Can you work these out from the model? Positions are in its coordinate system, mm. A direction names the side the tool comes from. Round coordinates to 2 decimals unless told otherwise and drop trailing zeros. Write each loop counter-clockwise with the first axis right and the second up, starting at its lowest first coordinate (ties: lowest second). Pieces come first, ordered by that corner, then holes. Notation, with made-up numbers: M -30.5,29 L -0.5,29 A26 ccw -0.5,57 Z; hole C 40,41.25 d9. An arc over 180 degrees is marked long. Answer as a JSON object with one key per item and string values. Group by question number.
1) Suppose I cut it at C-C, the plane y = 19. Write out the boundary of the cut face in (x, z).
2) Suppose I cut it at D-D, the plane x = 206. Write out the boundary of the cut face in (y, z).
3) I'm going to push flat-ended pins straight in: pin 1 Ø6 at (y, z) = (6, -75) entering from -X; pin 2 Ø8 at (x, y) = (156, 4) entering from +Z. Where does each tip first touch, or does it pass through?
4) Please list where these lines run through material, in increasing order: L1, parallel to X at y = 7.75, z = -46; L2, parallel to Z at x = 6.5, y = 6; L3, parallel to Y at x = 6, z = -75. Write a range as [from, to].
5) On a 3-axis mill with a long thin cutter (end or side, diameter ignored), from which of +Z, -Z, +X, -X, +Y, -Y can I reach the whole of each face in a straight line? I mean faces 1 (the flat face through (109, 11, -141)), 2 (the flat face through (109, 26, -121.5)), 3 (the flat face through (109, 28.67, -123)). Say none if no direction works.
6) Suppose I cut it at A-A, the plane x = 70. Write out the boundary of the cut face in (y, z).
7) Suppose I cut it at B-B, the plane z = -100. Write out the boundary of the cut face in (x, y), and give its area (3 significant figures).
8) If we mould it in two halves opening along Z, with no side actions, what happens to faces 4 (the flat face through (109, 12, -150)), 5 (the flat face through (0, 12, -72)), 6 (the flat face through (109, 23, 0)), 7 (the flat face through (193.5, 26, -70))? For each: +Z half, -Z half, draft (parallel to the pull), parting line (faces both ways), or undercut.
from build123d import *

# Parameters (mm, degrees)
BOSS_EXTRUDE1_DEPTH                               = 22.59
SKETCH2_W                                         = 220
SKETCH2_H                                         = 150
SKETCH2_W_2                                       = 167
SKETCH2_H_2                                       = 102
BOSS_EXTRUDE2_DEPTH                               = 6.08
CSK_FOR_6_FLAT_HEAD_SOCKET_CAP_SCREW2_D           = 3.7973
CSK_FOR_6_FLAT_HEAD_SOCKET_CAP_SCREW2_DEPTH       = 9
CSK_FOR_6_FLAT_HEAD_SOCKET_CAP_SCREW2_CSINK_D     = 7.7978
CSK_FOR_6_FLAT_HEAD_SOCKET_CAP_SCREW2_CSINK_ANGLE = 82
CSK_FOR_6_FLAT_HEAD_SOCKET_CAP_SCREW3_D           = 3.7973
CSK_FOR_6_FLAT_HEAD_SOCKET_CAP_SCREW3_CSINK_D     = 7.7978
CSK_FOR_6_FLAT_HEAD_SOCKET_CAP_SCREW3_CSINK_ANGLE = 82
CSK_FOR_6_FLAT_HEAD_SOCKET_CAP_SCREW4_D           = 3.7973
CSK_FOR_6_FLAT_HEAD_SOCKET_CAP_SCREW4_CSINK_D     = 7.7978
CSK_FOR_6_FLAT_HEAD_SOCKET_CAP_SCREW4_CSINK_ANGLE = 82
FILLET1_R                                         = 4


with BuildPart() as part:
    # Sketch1 → Boss-Extrude1 (new body)
    with BuildSketch(Plane(origin=(0, 0, 0), x_dir=(1, 0, 0), z_dir=(0, 1, 0))):
        Polygon((211, 0), (220, 0), (220, 150), (0, 150), (0, 0), (9, 0), (9, 141), (211, 141), align=None)
    extrude(amount=BOSS_EXTRUDE1_DEPTH)

    # Sketch2 → Boss-Extrude2 (add)
    with BuildSketch(Plane(origin=(0, 22.59, 0), x_dir=(1, 0, 0), z_dir=(0, 1, 0))):
        with Locations((110, 75)):
            Rectangle(SKETCH2_W, SKETCH2_H)
        with Locations((110, 70.5)):
            Rectangle(SKETCH2_W_2, SKETCH2_H_2, mode=Mode.SUBTRACT)
    extrude(amount=BOSS_EXTRUDE2_DEPTH)

    # CSK for #6 Flat Head Socket Cap Screw2
    with Locations(Plane(origin=(220, 0, 0), x_dir=(0, 0, -1), z_dir=(1, 0, 0))):
        with Locations((75, 6)):
            CounterSinkHole(CSK_FOR_6_FLAT_HEAD_SOCKET_CAP_SCREW2_D / 2, CSK_FOR_6_FLAT_HEAD_SOCKET_CAP_SCREW2_CSINK_D / 2, depth=CSK_FOR_6_FLAT_HEAD_SOCKET_CAP_SCREW2_DEPTH, counter_sink_angle=CSK_FOR_6_FLAT_HEAD_SOCKET_CAP_SCREW2_CSINK_ANGLE)

    # CSK for #6 Flat Head Socket Cap Screw3 (through all)
    with Locations(Plane(origin=(0, 0, -150), x_dir=(-1, 0, 0), z_dir=(0, 0, -1))):
        with Locations((-110, 6)):
            CounterSinkHole(CSK_FOR_6_FLAT_HEAD_SOCKET_CAP_SCREW3_D / 2, CSK_FOR_6_FLAT_HEAD_SOCKET_CAP_SCREW3_CSINK_D / 2, counter_sink_angle=CSK_FOR_6_FLAT_HEAD_SOCKET_CAP_SCREW3_CSINK_ANGLE)

    # CSK for #6 Flat Head Socket Cap Screw4 (through all)
    with Locations(Plane.ZY):
        with Locations((-75, 6)):
            CounterSinkHole(CSK_FOR_6_FLAT_HEAD_SOCKET_CAP_SCREW4_D / 2, CSK_FOR_6_FLAT_HEAD_SOCKET_CAP_SCREW4_CSINK_D / 2, counter_sink_angle=CSK_FOR_6_FLAT_HEAD_SOCKET_CAP_SCREW4_CSINK_ANGLE)

    # Fillet1
    fillet1_edges = [part.edges().sort_by_distance(p)[0] for p in [
        (0, 14.335, -150),
        (220, 14.335, -150),
        (0, 28.67, -75),
        (220, 28.67, -75),
        (110, 28.67, -150),
    ]]
    fillet(fillet1_edges, radius=FILLET1_R)


solid = part.part
Results:
{
 "1": {"outline": "M 0,-146 A4 ccw 4,-150 L 216,-150 A4 ccw 220,-146 L 220,0 L 211,0 L 211,-141 L 9,-141 L 9,0 L 0,0 Z"},
 "2": {"outline": "M 0,-150 L 24.67,-150 A4 ccw 28.67,-146 L 28.67,0 L 22.59,0 L 22.59,-141 L 0,-141 Z"},
 "3": {"pin 1": "x = 1.03", "pin 2": "z = -141"},
 "4": {"L1": "[0, 9], [211, 220]", "L2": "[-150, -76.9], [-73.1, 0]", "L3": "[0, 4.1], [7.9, 28.67]"},
 "5": {"face 1": "+Z, -Y", "face 2": "+Y, -Y", "face 3": "+Z, -Z, +X, -X, +Y"},
 "6": {"outline": "M 0,-150 L 24.67,-150 A4 ccw 28.67,-146 L 28.67,-121.5 L 22.59,-121.5 L 22.59,-141 L 0,-141 Z; M 22.59,-19.5 L 28.67,-19.5 L 28.67,0 L 22.59,0 Z"},
 "7": {"outline": "M 0,0 L 9,0 L 9,22.59 L 26.5,22.59 L 26.5,28.67 L 4,28.67 A4 ccw 0,24.67 Z; M 193.5,22.59 L 211,22.59 L 211,0 L 220,0 L 220,24.67 A4 ccw 216,28.67 L 193.5,28.67 Z", "area": "722 mm^2"},
 "8": {"face 4": "-Z half", "face 5": "draft", "face 6": "+Z half", "face 7": "undercut"}
}
